Could you check a few things on this model? Use its own coordinates, in mm. Face numbers are marked on the shaded views. A direction names the side the tool comes from. Give positions to 0.01 mm unless a question says otherwise; leave off trailing zeros. Loops run counter-clockwise (first coordinate to the right, second up) from the corner with the lowest first, then second, coordinate; pieces in that order, holes last. Notation, with made-up numbers: M -5.75,84.25 L 25.25,84.25 A19 cw 25.25,105.25 Z; hole C 24,-10.5 d11. An arc over 180 degrees is marked long. Return JSON: item names as keys, results as strings. Group by question number.
1. If we section it at A-A (x = 37.5): Write out the boundary of the cut face in (y, z), plus the area to 3 significant figures.
2. If we mould it in two halves opening along X, with no side actions, what happens to the marked faces 1, 2 and 3? For each: +X half, -X half, draft (parallel to the pull), parting line (faces both ways), or undercut.
3. If we section it at C-C (z = 9): Write out the boundary of the cut face in (x, y), plus the area to 3 significant figures.
4. For the marked faces 4 and 5, which set-ups out of +Z, -Z, +X, -X, +Y, -Y let a thin tool reach every point of the face, with its end or its side?
5. Please list where these lines run through material, in increasing order: line 1 (Y direction, x = 37.5, z = 14.05); line 2 (X direction, y = -9, z = 2.25); line 3 (Y direction, x = 37.5, z = 9).
6. If we section it at B-B (y = -10.5): Write out the boundary of the cut face in (x, z).
7. For pin 1 (2.5 mm diameter, centred on x = 9.5, y = -10.5, fed in from +Z), with a flat end and sliding along its axis, tell me the tip position at first contact or that it passes through.
8. If we section it at D-D (y = -7.75): Write out the boundary of the cut face in (x, z), plus the area to 3 significant figures.
```python
from build123d import *

# Parameters (mm, degrees)
F1_DEPTH = 21
F2_R     = 5
F4_DEPTH = 25
F5_R     = 3
F6_R     = 4.5
F7_DEPTH = 4


with BuildPart() as f1:
    # F0 (on Front) → F1 (new body)
    with BuildSketch(Plane.XZ):
        Polygon((55.5, 17), (6.891753, 17), (0, 17), (0, 0), (55.5, 0), align=None)
    extrude(amount=F1_DEPTH)

    # F2
    f2_edges = [f1.edges().sort_by_distance(p)[0] for p in [
        (55.5, -10.5, 17),
    ]]
    fillet(f2_edges, radius=F2_R)

    # F3 (on face) → F4 (cut)
    with BuildSketch(Plane.XY.offset(17)):
        with BuildLine():
            ThreePointArc((39.5, -10.5), (37.5, -8.5), (35.5, -10.5))
            Line((35.5, -10.5), (39.5, -10.5))
        make_face()
        with BuildLine():
            Line((39.5, -10.5), (35.5, -10.5))
            ThreePointArc((35.5, -10.5), (37.5, -12.5), (39.5, -10.5))
        make_face()
        with BuildLine():
            ThreePointArc((7.75, -10.5), (9.75, -12.5), (11.75, -10.5))
            Line((11.75, -10.5), (7.75, -10.5))
        make_face()
        with BuildLine():
            Line((7.75, -10.5), (11.75, -10.5))
            ThreePointArc((11.75, -10.5), (9.75, -8.5), (7.75, -10.5))
        make_face()
    extrude(amount=-F4_DEPTH, mode=Mode.SUBTRACT)

    # F5
    f5_edges = [f1.edges().sort_by_distance(p)[0] for p in [
        (0, -10.5, 17),
    ]]
    fillet(f5_edges, radius=F5_R)

    # F6 (on face) → F7 (cut)
    with BuildSketch(Plane.XY.offset(17)):
        with Locations((9.75, -10.5)):
            Circle(F6_R)
        with Locations((37.5, -10.5)):
            Circle(F6_R)
    extrude(amount=-F7_DEPTH, mode=Mode.SUBTRACT)


solid = f1.part
```
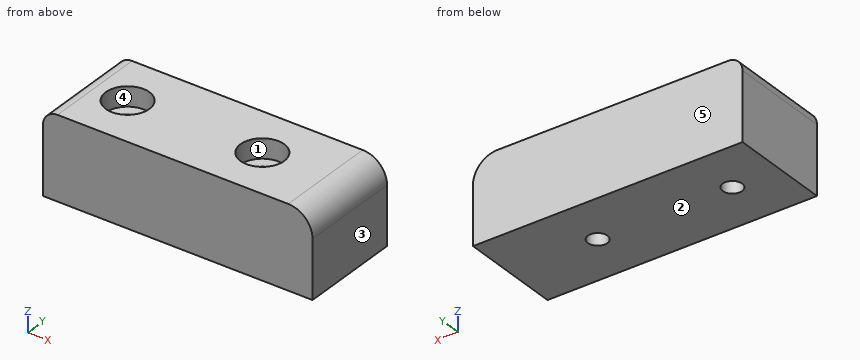
Answer:
{
 "1": {"outline": "M -21,0 L -12.5,0 L -12.5,13 L -15,13 L -15,17 L -21,17 Z; M -8.5,0 L 0,0 L 0,17 L -6,17 L -6,13 L -8.5,13 Z", "area": "269 mm²"},
 "2": {"face 1": "undercut", "face 2": "draft", "face 3": "+X half"},
 "3": {"outline": "M 0,-21 L 55.5,-21 L 55.5,0 L 0,0 Z; hole C 9.75,-10.5 d4; hole C 37.5,-10.5 d4", "area": "1,140 mm²"},
 "4": {"face 4": "+Z", "face 5": "+Z, -Z, +X, -X, +Y"},
 "5": {"line 1": "y = -21 to -15, -6 to 0", "line 2": "x = 0 to 8.43, 11.07 to 36.18, 38.82 to 55.5", "line 3": "y = -21 to -12.5, -8.5 to 0"},
 "6": {"outline": "M 0,0 L 7.75,0 L 7.75,13 L 5.25,13 L 5.25,17 L 3,17 A3 ccw 0,14 Z; M 11.75,0 L 35.5,0 L 35.5,13 L 33,13 L 33,17 L 14.25,17 L 14.25,13 L 11.75,13 Z; M 39.5,0 L 55.5,0 L 55.5,12 A5 ccw 50.5,17 L 42,17 L 42,13 L 39.5,13 Z"},
 "7": {"pin 1": "passes through"},
 "8": {"outline": "M 0,0 L 55.5,0 L 55.5,12 A5 ccw 50.5,17 L 41.06,17 L 41.06,13 L 33.94,13 L 33.94,17 L 13.31,17 L 13.31,13 L 6.19,13 L 6.19,17 L 3,17 A3 ccw 0,14 Z", "area": "879 mm²"}
}
